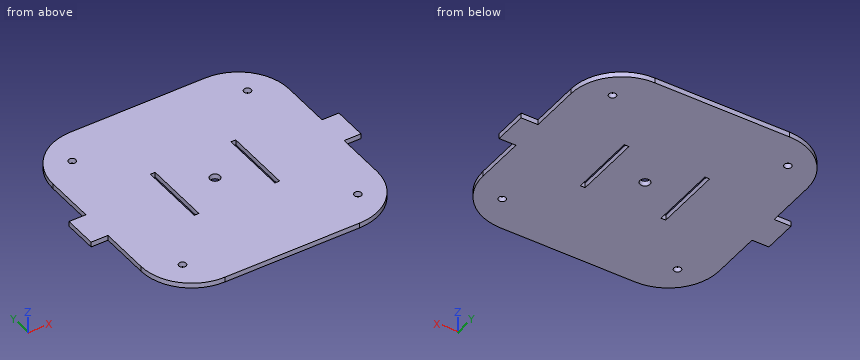
```python
from build123d import *

# Parameters (mm, degrees)
CROQUIS2_R              = 2.95
CROQUIS2_R_2            = 2.15
SALIENTE_EXTRUIR2_DEPTH = 3


with BuildPart() as part:
    # Croquis2 → Saliente-Extruir2 (new body)
    with BuildSketch(Plane.XY):
        with BuildLine():
            Line((30, 110), (110, 110))
            ThreePointArc((110, 110), (131.213203436, 101.213203436), (140, 80))
            Line((140, 80), (140, 50))
            Line((140, 50), (150, 50))
            Line((150, 50), (150, 40))
            Line((150, 40), (150, 30))
            Line((150, 30), (140, 30))
            Line((140, 30), (140, 0))
            ThreePointArc((140, 0), (131.213203436, -21.213203436), (110, -30))
            Line((110, -30), (30, -30))
            ThreePointArc((30, -30), (8.786796564, -21.213203436), (0, 0))
            Line((0, 0), (0, 30))
            Line((0, 30), (-10, 30))
            Line((-10, 30), (-10, 40))
            Line((-10, 40), (-10, 50))
            Line((-10, 50), (0, 50))
            Line((0, 50), (0, 80))
            ThreePointArc((0, 80), (8.786796564, 101.213203436), (30, 110))
        make_face()
        with Locations((70, 40)):
            Circle(CROQUIS2_R, mode=Mode.SUBTRACT)
        with Locations((18.016709675, -10)):
            Circle(CROQUIS2_R_2, mode=Mode.SUBTRACT)
        with Locations(Location((18.016709675, 90, 0), (0, 0, 180))):
            Circle(CROQUIS2_R_2, mode=Mode.SUBTRACT)
        with Locations(Location((121.983290325, -10, 0), (0, 0, 180))):
            Circle(CROQUIS2_R_2, mode=Mode.SUBTRACT)
        with Locations((121.983290325, 90)):
            Circle(CROQUIS2_R_2, mode=Mode.SUBTRACT)
        Polygon((44.7, 59.85), (47.5, 59.85), (47.5, 40), (47.5, 20.15), (44.7, 20.15), align=None, mode=Mode.SUBTRACT)
        Polygon((92.5, 59.85), (92.5, 40), (92.5, 20.15), (95.3, 20.15), (95.3, 59.85), align=None, mode=Mode.SUBTRACT)
    extrude(amount=SALIENTE_EXTRUIR2_DEPTH)


solid = part.part
```
Design review of the part built by this model. Coordinates are the model's own, in mm. Coordinates: 2 decimals unless noted, no trailing zeros. Loops run counter-clockwise (first coordinate to the right, second up) from the corner with the lowest first, then second, coordinate; pieces in that order, holes last. Notation, with made-up numbers: M -21.5,67 L 17.5,67 A15 ccw 17.5,87 Z; hole C 59,28 d7. An arc over 180 degrees is marked long. One line per question, with ' | ' between items.
(1) We need section C-C (z = 1.75). Count the separate pieces of the cut face and the enclosed holes in it, and give its area (3 significant figures).
Filled in:
separate pieces: 1 | enclosed holes: 7 | area: 18,900 mm^2
(2) We need section D-D (y = 90). Give the boundary of the cut face in (x, z).
Filled in:
outline: M 1.72,0 L 15.87,0 L 15.87,3 L 1.72,3 Z; M 20.17,0 L 119.83,0 L 119.83,3 L 20.17,3 Z; M 124.13,0 L 138.28,0 L 138.28,3 L 124.13,3 Z
(3) We need section A-A (y = 32.5). Give the boundary of the cut face in (x, z).
Filled in:
outline: M -10,0 L 44.7,0 L 44.7,3 L -10,3 Z; M 47.5,0 L 92.5,0 L 92.5,3 L 47.5,3 Z; M 95.3,0 L 150,0 L 150,3 L 95.3,3 Z
(4) We need section B-B (x = 70). Give the boundary of the cut face in (y, z), and give its area (3 significant figures).
Filled in:
outline: M -30,0 L 37.05,0 L 37.05,3 L -30,3 Z; M 42.95,0 L 110,0 L 110,3 L 42.95,3 Z | area: 402 mm^2
(5) Wall thickness on probe 1 along X at (y, z) = (59, 1.75); probe 2 along X at (y, z) = (41, 1.95); probe 3 along Y at (x, z) = (94, 1.5): over which ranges is each line inside the solid? List them lowest first.
Filled in:
probe 1: x = 0 to 44.7, 47.5 to 92.5, 95.3 to 140 | probe 2: x = -10 to 44.7, 47.5 to 67.22, 72.78 to 92.5, 95.3 to 150 | probe 3: y = -30 to 20.15, 59.85 to 110
(6) For pin 1 Ø0.9 at (y, z) = (60, 1.5) entering from -X; pin 2 Ø0.9 at (x, z) = (-5, 1) entering from +Y; pin 3 Ø0.9 at (y, z) = (59, 2) entering from +X, all flat-tipped, find the tip position at first contact; note any pin that passes through.
Filled in:
pin 1: stops at x = 0 | pin 2: stops at y = 50 | pin 3: stops at x = 140
